The figure shows three views and two pictorial views of one solid part (mm, origin at its lowest corner). Answer the questions. A direction names the side the tool comes from. Coordinates: 2 decimals unless noted, no trailing zeros. Order: outer loops, then holes, each group sorted by start corner. A loop starts at its lowest first (then second) coordinate and runs counter-clockwise, first axis right, second up. Notation, with made-up numbers: M -11,-21 L -1,-21 A10 cw -1,-16 Z; hole C 42,9.25 d7. An arc over 180 degrees is marked long. Write item = value, one per line. Start each with the question number.
Q1. Straight lines are drawn through the part: line 1 along Z through (x, y) = (41, 14.5); line 2 along Y through (x, z) = (30, 15.5). For each, find the intervals that lie inside material, in ascending order.
Q2. A tool of negligible diameter and unlimited length cuts with its end or side. For the marked faces 4 and 5, from which of +Z, -Z, +X, -X, +Y, -Y can it reach the whole face along a straight path? Write none if from no direction.
Q3. Find section C-C on z = 27. Give the vertices of the cut face in (x, y), and give its area (3 significant figures).
Q4. Determine the mould class of the marked faces 1, 2 and 3 for opening direction Z: released by +Z, released by -Z, zero draft, split by the parting line, or undercut.
Q5. Find section A-A on y = 3.5. Give the vertices of the cut face in (x, z).
Q6. This flat-tipped pin is pushed along its axis until it touches: P1, Ø10, axis at x = 28, z = 23, coming from the -Y side. Where does it stop, or does it pass through?
Q7. Find section B-B on x = 41.5. Give the vertices of the cut face in (y, z), and give its area (3 significant figures).
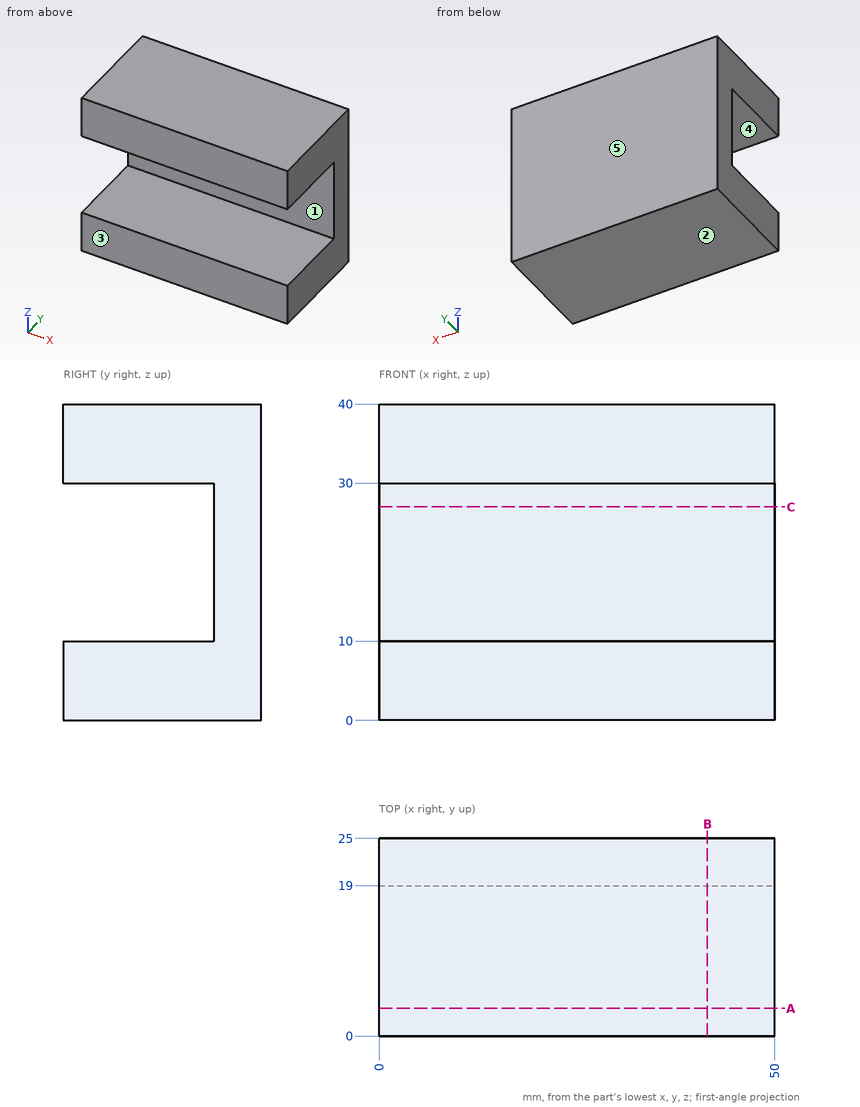
Findings below:
q1.line_1 = 0 to 10, 30 to 40
q1.line_2 = 19 to 25
q2.face_4 = +X, -X, -Y
q2.face_5 = +Z, -Z, +X, -X, +Y
q3.outline = M 0,19 L 50,19 L 50,25 L 0,25 Z
q3.area = 300 mm^2
q4.face_1 = undercut
q4.face_2 = released by -Z
q4.face_3 = zero draft
q5.outline = M 0,0 L 50,0 L 50,10 L 0,10 Z; M 0,30 L 50,30 L 50,40 L 0,40 Z
q6.P1 = 19
q7.outline = M 0,0 L 25,0 L 25,40 L 0,40 L 0,30 L 19,30 L 19,10 L 0,10 Z
q7.area = 620 mm^2
